```python
from build123d import *

# Parameters (mm, degrees)
SKETCH1_R           = 12.5
BOSS_EXTRUDE1_DEPTH = 31.75
SKETCH2_R           = 1
BOSS_EXTRUDE2_DEPTH = 10
SKETCH3_R           = 1.5
CUT_EXTRUDE1_DEPTH  = 6.35


with BuildPart() as part:
    # Sketch1 → Boss-Extrude1 (new body)
    with BuildSketch(Plane(origin=(0, 0, 0), x_dir=(1, 0, 0), z_dir=(0, 1, 0))):
        with Locations(Location((0, 0, 0), (0, 0, 270))):
            Circle(SKETCH1_R)
    extrude(amount=BOSS_EXTRUDE1_DEPTH)

    # Sketch2 → Boss-Extrude2 (add)
    with BuildSketch(Plane(origin=(0, 31.75, 0), x_dir=(1, 0, 0), z_dir=(0, 1, 0))):
        with Locations(Location((0, 0, 0), (0, 0, 270))):
            Circle(SKETCH2_R)
    extrude(amount=BOSS_EXTRUDE2_DEPTH)

    # Sketch3 → Cut-Extrude1 (cut)
    with BuildSketch(Plane(origin=(0, 31.75, 0), x_dir=(1, 0, 0), z_dir=(0, 1, 0))):
        with Locations(Location((-8.5, 0, 0), (0, 0, 270))):
            Circle(SKETCH3_R)
        with Locations(Location((8.5, 0, 0), (0, 0, 270))):
            Circle(SKETCH3_R)
    extrude(amount=-CUT_EXTRUDE1_DEPTH, mode=Mode.SUBTRACT)


solid = part.part
```
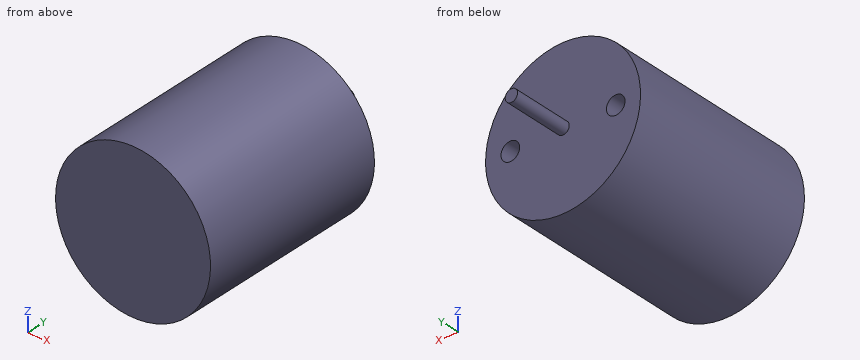
Design review of the part built by this model. Coordinates are the model's own, in mm. Coordinates: 2 decimals unless noted, no trailing zeros. Order: outer loops, then holes, each group sorted by start corner. A loop starts at its lowest first (then second) coordinate and runs counter-clockwise, first axis right, second up.
1) Take a section at D-D, the plane x = -9. Give the boundary of the cut face in (y, z), and give its area (3 significant figures).
2) Take a section at A-A, the plane x = 0. Give the boundary of the cut face in (y, z).
3) Take a section at C-C, the plane y = 36. Give the boundary of the cut face in (x, z).
4) Wall thickness on line 1 along X through (y, z) = (28.75, 0); line 2 along Y through (x, z) = (-4.5, -4.5); line 3 along Y through (x, z) = (8.75, 1): over which ranges is each line inside the solid? List them lowest first.
5) Clearance check with flat-ended pins moving along their axes: pin 1 (5 mm diameter, centred on x = 8.5, z = 0, fed in from -Y); pin 2 (0.9 mm diameter, centred on x = -9, z = -0.5, fed in from +Y); pin 3 (6 mm diameter, centred on y = 34, z = -7, fed in from -X); pin 4 (1.5 mm diameter, centred on x = -2.5, y = 4.5, fed in from -Z). State where each tip first meets the part, or that it passes through.
6) Take a section at B-B, the plane z = 0. Give the boundary of the cut face in (x, y).
Returned:
1. outline: (0, -8.67) - (31.75, -8.67) - (31.75, -1.41) - (25.4, -1.41) - (25.4, 1.41) - (31.75, 1.41) - (31.75, 8.67) - (0, 8.67) - close
1. area: 533 mm2
2. outline: (0, -12.5) - (31.75, -12.5) - (31.75, -1) - (41.75, -1) - (41.75, 1) - (31.75, 1) - (31.75, 12.5) - (0, 12.5) - close
3. outline: circle Ø2 at (0, 0)
4. line 1: x = -12.5 to -10, -7 to 7, 10 to 12.5
4. line 2: y = 0 to 31.75
4. line 3: y = 0 to 25.4
5. pin 1: stops at y = 0
5. pin 2: stops at y = 25.4
5. pin 3: stops at x = -11.45
5. pin 4: stops at z = -12.38
6. outline: (-12.5, 0) - (12.5, 0) - (12.5, 31.75) - (10, 31.75) - (10, 25.4) - (7, 25.4) - (7, 31.75) - (1, 31.75) - (1, 41.75) - (-1, 41.75) - (-1, 31.75) - (-7, 31.75) - (-7, 25.4) - (-10, 25.4) - (-10, 31.75) - (-12.5, 31.75) - close
